from build123d import *

# Parameters (mm, degrees)
F0_R     = 1.8288
F0_R_2   = 1.5875
F1_DEPTH = 1.70942


with BuildPart() as f1:
    # F0 (on Top) → F1 (new body)
    with BuildSketch(Plane.XY):
        with BuildLine():
            Line((16.542796, 27.770879), (-16.542796, 27.770879))
            ThreePointArc((-16.542796, 27.770879), (-17.775421, 27.608601), (-18.924046, 27.132825))
            Line((-18.924046, 27.132825), (-40.921091, 14.432825))
            ThreePointArc((-40.921091, 14.432825), (-43.215428, 11.214078), (-42.288939, 7.371431))
            Line((-42.288939, 7.371431), (-22.822177, -17.478448))
            ThreePointArc((-22.822177, -17.478448), (-21.158047, -18.823358), (-19.073079, -19.304))
            Line((-19.073079, -19.304), (19.073079, -19.304))
            ThreePointArc((19.073079, -19.304), (21.158047, -18.823358), (22.822177, -17.478448))
            Line((22.822177, -17.478448), (42.288939, 7.371431))
            ThreePointArc((42.288939, 7.371431), (43.215428, 11.214078), (40.921091, 14.432825))
            Line((40.921091, 14.432825), (18.924046, 27.132825))
            ThreePointArc((18.924046, 27.132825), (17.775421, 27.608601), (16.542796, 27.770879))
        make_face()
        with Locations((-19.073079, -14.5415)):
            Circle(F0_R, mode=Mode.SUBTRACT)
        with Locations((19.073079, -14.5415)):
            Circle(F0_R, mode=Mode.SUBTRACT)
        with Locations((-38.539841, 10.308379)):
            Circle(F0_R_2, mode=Mode.SUBTRACT)
        with Locations((-16.542796, 23.008379)):
            Circle(F0_R_2, mode=Mode.SUBTRACT)
        with Locations((38.539841, 10.308379)):
            Circle(F0_R_2, mode=Mode.SUBTRACT)
        with Locations((16.542796, 23.008379)):
            Circle(F0_R_2, mode=Mode.SUBTRACT)
    extrude(amount=F1_DEPTH)


solid = f1.part
Verification items for the finished model (mm, model axes). Round coordinates to 2 decimals unless told otherwise and drop trailing zeros. Loops run counter-clockwise (first coordinate to the right, second up) from the corner with the lowest first, then second, coordinate; pieces in that order, holes last. Notation, with made-up numbers: (-39, 41) - (12, 41) arc R21 cw to (12, 50) - close; hole circle Ø6 at (-19.75, -3.5). An arc over 180 degrees is marked (long way). Answer in a Markdown table with one row per item. Add a question column.
Q1. Material ranges on line 1 (Y direction, x = 18, z = 0.45); line 2 (X direction, y = 11, z = 1.55); line 3 (Y direction, x = -39.5, z = 0.7), recorded low to high.
Q2. Section check A-A on z = 1.4. Enter the section's corners in (x, y) (1 decimal).
Q3. Section check B-B on y = -10.5. Enter the section's corners in (x, z), plus the area to 3 significant figures.
Q4. Section check C-C on y = -2. Enter the section's corners in (x, z).
Found:
| question | item | result |
|---|---|---|
| 1 | line 1 | y = -19.3 to -16.02, -13.06 to 22.38, 23.64 to 27.54 |
| 1 | line 2 | x = -43.25 to -39.97, -37.11 to 37.11, 39.97 to 43.25 |
| 1 | line 3 | y = 3.81 to 9.04, 11.57 to 15.25 |
| 2 | outline | (-42.3, 7.4) - (-22.8, -17.5) arc R4.8 ccw to (-19.1, -19.3) - (19.1, -19.3) arc R4.8 ccw to (22.8, -17.5) - (42.3, 7.4) arc R4.8 ccw to (40.9, 14.4) - (18.9, 27.1) arc R4.8 ccw to (16.5, 27.8) - (-16.5, 27.8) arc R4.8 ccw to (-18.9, 27.1) - (-40.9, 14.4) arc R4.8 ccw to start; hole circle Ø3.2 at (-38.5, 10.3); hole circle Ø3.7 at (-19.1, -14.5); hole circle Ø3.2 at (-16.5, 23); hole circle Ø3.2 at (16.5, 23); hole circle Ø3.7 at (19.1, -14.5); hole circle Ø3.2 at (38.5, 10.3) |
| 3 | outline | (-28.29, 0) - (28.29, 0) - (28.29, 1.71) - (-28.29, 1.71) - close |
| 3 | area | 96.7 mm² |
| 4 | outline | (-34.95, 0) - (34.95, 0) - (34.95, 1.71) - (-34.95, 1.71) - close |
